Verification items for the finished model (mm, model axes). Face numbers are marked on the shaded views. A direction names the side the tool comes from. Give positions to 0.01 mm unless a question says otherwise; leave off trailing zeros. Loops run counter-clockwise (first coordinate to the right, second up) from the corner with the lowest first, then second, coordinate; pieces in that order, holes last. Notation, with made-up numbers: M 83.5,77 L 130.5,77 A10 ccw 130.5,86 Z; hole C -30,1 d5. An arc over 180 degrees is marked long. Put each result on its own line as item: value. Start each with the question number.
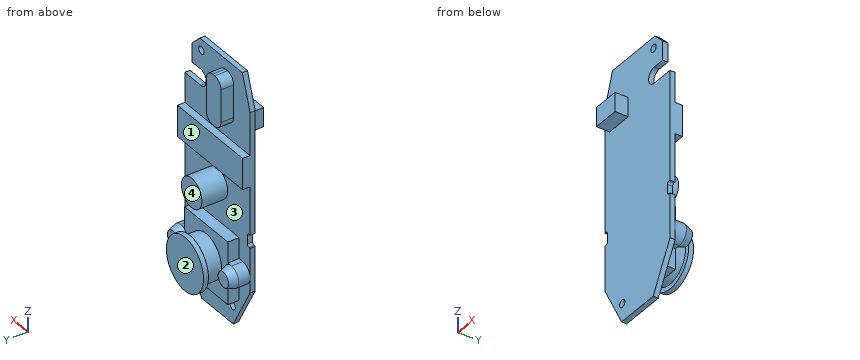
from build123d import *

# Parameters (mm, degrees)
SKETCH_1_R      = 0.85
EXTRUDE_1_DEPTH = 1.15
EXTRUDE_2_DEPTH = 2.54
SKETCH_3_R      = 4.95
EXTRUDE_3_DEPTH = 3.65
SKETCH_4_R      = 5.985
EXTRUDE_4_DEPTH = 1.1
SKETCH_5_R      = 2.35
EXTRUDE_5_DEPTH = 1.825
EXTRUDE_5_TAPER = 20
SKETCH_6_R      = 3.3
EXTRUDE_6_DEPTH = 5.8
SKETCH_7_W      = 21.05
SKETCH_7_H      = 7
EXTRUDE_7_DEPTH = 1.65
EXTRUDE_8_DEPTH = 2.85
SKETCH_9_W      = 6
SKETCH_9_H      = 4.3
EXTRUDE_9_DEPTH = 2.95


with BuildPart() as part:
    # Эскиз1 → Бобышка-Вытянуть1 (new body)
    with BuildSketch(Plane(origin=(0, 0, 0), x_dir=(1, 0, 0), z_dir=(0, 1, 0))):
        with BuildLine():
            Line((5.1, 17.801195131), (10.525, 7.801195131))
            Line((10.525, 7.801195131), (10.525, -2.198804869))
            Line((10.525, -2.198804869), (10.175, -2.198804869))
            ThreePointArc((10.175, -2.198804869), (9.821446609, -2.345251479), (9.675, -2.698804869))
            Line((9.675, -2.698804869), (9.675, -4.598804869))
            ThreePointArc((9.675, -4.598804869), (9.821446609, -4.95235826), (10.175, -5.098804869))
            Line((10.175, -5.098804869), (10.525, -5.098804869))
            Line((10.525, -5.098804869), (10.525, -29.618804869))
            Line((10.525, -29.618804869), (5.425, -29.618804869))
            ThreePointArc((5.425, -29.618804869), (3.625, -31.418804869), (5.425, -33.218804869))
            Line((5.425, -33.218804869), (8.175, -33.218804869))
            Line((8.175, -33.218804869), (8.175, -37.518804869))
            Line((8.175, -37.518804869), (5.675, -40.018804869))
            Line((5.675, -40.018804869), (-8.025, -40.018804869))
            Line((-8.025, -40.018804869), (-10.525, -32.518804869))
            Line((-10.525, -32.518804869), (-10.525, -5.098804869))
            Line((-10.525, -5.098804869), (-10.175, -5.098804869))
            ThreePointArc((-10.175, -5.098804869), (-9.821446609, -4.95235826), (-9.675, -4.598804869))
            Line((-9.675, -4.598804869), (-9.675, -2.698804869))
            ThreePointArc((-9.675, -2.698804869), (-9.821446609, -2.345251479), (-10.175, -2.198804869))
            Line((-10.175, -2.198804869), (-10.525, -2.198804869))
            Line((-10.525, -2.198804869), (-10.525, 7.801195131))
            Line((-10.525, 7.801195131), (-5.1, 17.801195131))
            Line((-5.1, 17.801195131), (5.1, 17.801195131))
        make_face()
        with Locations(Location((5.211720062, -37.568804869, 0), (0, 0, 270))):
            Circle(SKETCH_1_R, mode=Mode.SUBTRACT)
        with Locations(Location((-4.903634314, 13.801195131, 0), (0, 0, 270))):
            Circle(SKETCH_1_R, mode=Mode.SUBTRACT)
    extrude(amount=EXTRUDE_1_DEPTH)

    # Эскиз2 → Бобышка-Вытянуть2 (add)
    with BuildSketch(Plane(origin=(0, 1.15, 0), x_dir=(1, 0, 0), z_dir=(0, 1, 0))):
        with BuildLine():
            Line((-7, 11.421195131), (7, 11.421195131))
            Line((7, 11.421195131), (7, 6.797688136))
            Line((7, 6.797688136), (8.175, 6.797688136))
            ThreePointArc((8.175, 6.797688136), (10.525, 4.447688136), (8.175, 2.097688136))
            Line((8.175, 2.097688136), (7, 2.097688136))
            Line((7, 2.097688136), (7, -2.578804869))
            Line((7, -2.578804869), (-7, -2.578804869))
            Line((-7, -2.578804869), (-7, 2.097688136))
            Line((-7, 2.097688136), (-8.175, 2.097688136))
            ThreePointArc((-8.175, 2.097688136), (-10.525, 4.447688136), (-8.175, 6.797688136))
            Line((-8.175, 6.797688136), (-7, 6.797688136))
            Line((-7, 6.797688136), (-7, 11.421195131))
        make_face()
    extrude(amount=EXTRUDE_2_DEPTH)

    # Эскиз3 → Бобышка-Вытянуть3 (add)
    with BuildSketch(Plane(origin=(0, 3.69, 0), x_dir=(1, 0, 0), z_dir=(0, 1, 0))):
        with Locations(Location((0, 4.421195131, 0), (0, 0, 270))):
            Circle(SKETCH_3_R)
    extrude(amount=EXTRUDE_3_DEPTH)

    # Эскиз4 → Бобышка-Вытянуть4 (add)
    with BuildSketch(Plane(origin=(0, 7.34, 0), x_dir=(1, 0, 0), z_dir=(0, 1, 0))):
        with Locations(Location((0, 4.421195131, 0), (0, 0, 270))):
            Circle(SKETCH_4_R)
    extrude(amount=EXTRUDE_4_DEPTH)

    # Эскиз5 → Бобышка-Вытянуть5 (add)
    with BuildSketch(Plane(origin=(0, 3.69, 0), x_dir=(1, 0, 0), z_dir=(0, 1, 0))):
        with Locations((-8.175, 4.447688136)):
            Circle(SKETCH_5_R)
    extrude_5 = extrude(amount=EXTRUDE_5_DEPTH, taper=EXTRUDE_5_TAPER)

    # Зеркальное отражение1: Бобышка-Вытянуть5 across plane
    add(extrude_5.mirror(Plane(origin=(0, 0, 0), x_dir=(0, 0, 1), z_dir=(1, 0, 0))))

    # Эскиз6 → Бобышка-Вытянуть6 (add)
    with BuildSketch(Plane(origin=(0, 1.15, 0), x_dir=(1, 0, 0), z_dir=(0, 1, 0))):
        with Locations(Location((0, -10.898804869, 0), (0, 0, 270))):
            Circle(SKETCH_6_R)
    extrude(amount=EXTRUDE_6_DEPTH)

    # Эскиз7 → Бобышка-Вытянуть7 (add)
    with BuildSketch(Plane(origin=(0, 1.15, 0), x_dir=(1, 0, 0), z_dir=(0, 1, 0))):
        with Locations((0, -19.398804869)):
            Rectangle(SKETCH_7_W, SKETCH_7_H)
    extrude(amount=EXTRUDE_7_DEPTH)

    # Эскиз8 → Бобышка-Вытянуть8 (add)
    with BuildSketch(Plane(origin=(0, 1.15, 0), x_dir=(1, 0, 0), z_dir=(0, 1, 0))):
        with BuildLine():
            Line((-3.225, -26.418804869), (-2.525, -26.418804869))
            ThreePointArc((-2.525, -26.418804869), (-1.110786438, -27.004591307), (-0.525, -28.418804869))
            Line((-0.525, -28.418804869), (-0.525, -35.718804869))
            ThreePointArc((-0.525, -35.718804869), (-1.110786438, -37.133018432), (-2.525, -37.718804869))
            Line((-2.525, -37.718804869), (-3.225, -37.718804869))
            ThreePointArc((-3.225, -37.718804869), (-4.639213562, -37.133018432), (-5.225, -35.718804869))
            Line((-5.225, -35.718804869), (-5.225, -28.418804869))
            ThreePointArc((-5.225, -28.418804869), (-4.639213562, -27.004591307), (-3.225, -26.418804869))
        make_face()
    extrude(amount=EXTRUDE_8_DEPTH)

    # Эскиз9 → Бобышка-Вытянуть9 (add)
    with BuildSketch(Plane.XZ):
        with Locations((-5.975, 29.018804869)):
            Rectangle(SKETCH_9_W, SKETCH_9_H)
    extrude(amount=EXTRUDE_9_DEPTH)


solid = part.part
Q1. Cross-section at C-C, the plane y = 6.25. Record the boundary of the cut face in (x, z).
Q2. Scan lines: L1, parallel to Y at x = 7.25, z = 18.5; L2, parallel to X at y = 5.25, z = -6; L3, parallel to Y at x = 8.5, z = 10.5. Record each from-to range of solid material in increasing order.
Q3. Go/stop test with flat-tipped pins: pin 1 (1.3 mm diameter, centred on y = 2, z = -8, fed in from -X); pin 2 (1.3 mm diameter, centred on x = 4.5, y = 2, fed in from -Z); pin 3 (6.5 mm diameter, centred on x = -4, z = 14, fed in from -Y). Record where each tip stops, or that it passes through.
Q4. Cross-section at D-D, the plane z = 0. Record the boundary of the cut face in (x, y) (3 decimals).
Q5. Set-up check for the marked faces 3 and 4: record each of +Z, -Z, +X, -X, +Y, -Y from which the full face is reachable in a straight line by a thin tool's end or side.
Q6. Cross-section at B-B, the plane x = 0. Record the boundary of the cut face in (y, z), then the cut area to 3 significant figures.
Q7. Cross-section at A-A, the plane y = 2.25. Record the boundary of the cut face in (x, z) (3 decimals), then the cut area to 3 significant figures.
Q8. Release check for a two-part mould opening along Z. For the marked faces 1 and 2 record: pulls with the +Z half, pulls with the -Z half, needs draft (parallel to the pull), parting line crosses it, or undercut.
Ans:
1. outline: C 0,-4.42 d9.9; C 0,10.9 d6.6
2. L1: y = 0 to 2.8
2. L2: x = -9.05 to -7.3, -4.69 to 4.69, 7.3 to 9.05
2. L3: y = 0 to 1.15
3. pin 1: stops at x = -7
3. pin 2: stops at z = -11.42
3. pin 3: stops at y = 0
4. outline: M -10.525,0 L 10.525,0 L 10.525,1.15 L 7,1.15 L 7,3.69 L 2.226,3.69 L 2.226,7.34 L 4.034,7.34 L 4.034,8.44 L -4.034,8.44 L -4.034,7.34 L -2.226,7.34 L -2.226,3.69 L -7,3.69 L -7,1.15 L -10.525,1.15 Z
5. face 3: +Y
5. face 4: +Z, +X, -X, +Y
6. outline: M 0,-17.8 L 1.15,-17.8 L 1.15,-11.42 L 3.69,-11.42 L 3.69,-9.37 L 7.34,-9.37 L 7.34,-10.41 L 8.44,-10.41 L 8.44,1.56 L 7.34,1.56 L 7.34,0.53 L 3.69,0.53 L 3.69,2.58 L 1.15,2.58 L 1.15,7.6 L 6.95,7.6 L 6.95,14.2 L 1.15,14.2 L 1.15,15.9 L 2.8,15.9 L 2.8,22.9 L 1.15,22.9 L 1.15,40.02 L 0,40.02 Z
6. area: 201 mm^2
7. outline: M -10.525,15.899 L 10.525,15.899 L 10.525,22.899 L -10.525,22.899 Z; M -8.175,-6.798 L -7,-6.798 L -7,-11.421 L 7,-11.421 L 7,-6.798 L 8.175,-6.798 A2.35 ccw 8.175,-2.098 L 7,-2.098 L 7,2.579 L -7,2.579 L -7,-2.098 L -8.175,-2.098 A2.35 ccw Z; M -5.225,28.419 A2 ccw -3.225,26.419 L -2.525,26.419 A2 ccw -0.525,28.419 L -0.525,35.719 A2 ccw -2.525,37.719 L -3.225,37.719 A2 ccw -5.225,35.719 Z; C 0,10.899 d6.6
7. area: 456 mm^2
8. face 1: undercut
8. face 2: needs draft
